Check sheet for the drawn part. Datum: minimum x, y, z corner. Units: mm. Coordinates: 2 decimals unless noted, no trailing zeros. Write each loop counter-clockwise with the first axis right and the second up, starting at its lowest first coordinate (ties: lowest second). Pieces come first, ordered by that corner, then holes. Notation, with made-up numbers: (73.5, -39.75) - (114.5, -39.75) arc R19 ccw to (114.5, -6.75) - close; hole circle Ø3 at (15, 28.25). An arc over 180 degrees is marked (long way). Write each question's results on one line, items separated by ' | '.
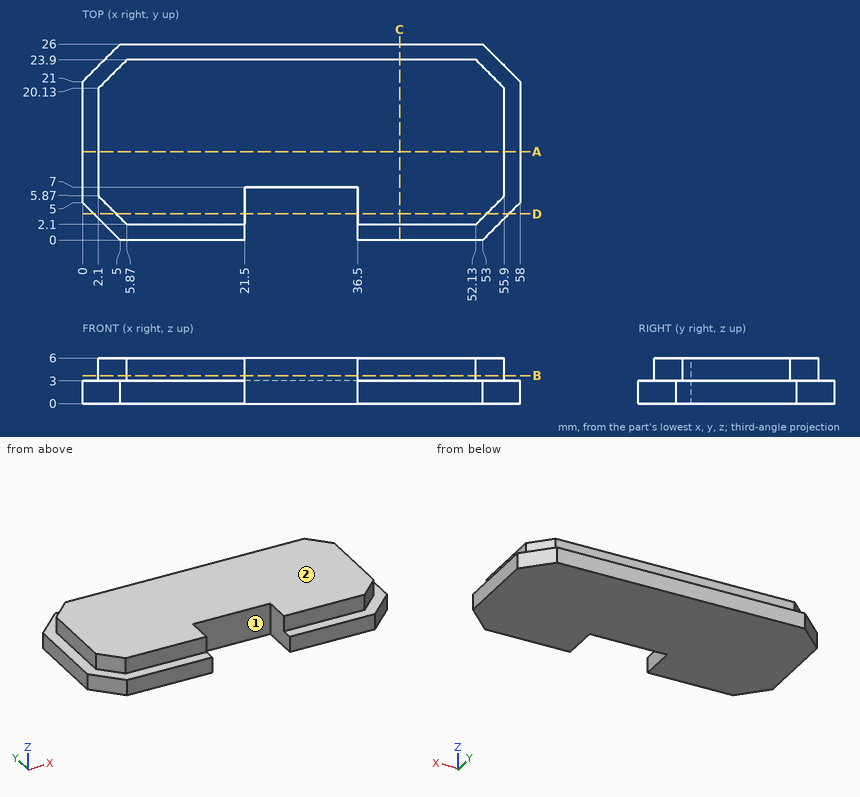
1. Draft check along X on the marked faces 1 and 2. Enter one of: pulls with the +X half, pulls with the -X half, needs draft (parallel to the pull), parting line crosses it, or undercut.
Values follow:
face 1: undercut | face 2: needs draft
2. Go/stop test with flat-tipped pins: pin 1 (0.9 mm diameter, centred on x = 23.5, z = 4, fed in from +Y); pin 2 (1 mm diameter, centred on y = 11, z = 5.5, fed in from +X); pin 3 (1.5 mm diameter, centred on y = 12.5, z = 5, fed in from -X). Record where each tip stops, or that it passes through.
Values follow:
pin 1: stops at y = 23.9 | pin 2: stops at x = 55.9 | pin 3: stops at x = 2.1
3. Sectioned sample at D-D (y = 3.5). Record the cut outline in (x, z), then the cut area to 3 significant figures.
Values follow:
outline: (1.5, 0) - (21.5, 0) - (21.5, 6) - (4.47, 6) - (4.47, 3) - (1.5, 3) - close; (36.5, 0) - (56.5, 0) - (56.5, 3) - (53.53, 3) - (53.53, 6) - (36.5, 6) - close | area: 222 mm^2
4. Material ranges on L1, parallel to X at y = 5.5, z = 2.3; L2, parallel to X at y = 14.25, z = 3.4; L3, parallel to Z at x = 8.5, y = 1.75, recorded low to high. Write a range as [from, to].
Values follow:
L1: x = [0, 21.5], [36.5, 58] | L2: x = [2.1, 55.9] | L3: z = [0, 3]
5. Sectioned sample at A-A (y = 11.75). Record the cut outline in (x, z), then the cut area to 3 significant figures.
Values follow:
outline: (0, 0) - (58, 0) - (58, 3) - (55.9, 3) - (55.9, 6) - (2.1, 6) - (2.1, 3) - (0, 3) - close | area: 335 mm^2
6. Sectioned sample at C-C (x = 42). Record the cut outline in (y, z).
Values follow:
outline: (0, 0) - (26, 0) - (26, 3) - (23.9, 3) - (23.9, 6) - (2.1, 6) - (2.1, 3) - (0, 3) - close
7. Sectioned sample at B-B (z = 3.7). Record the cut outline in (x, y).
Values follow:
outline: (2.1, 5.87) - (5.87, 2.1) - (21.5, 2.1) - (21.5, 7) - (36.5, 7) - (36.5, 2.1) - (52.13, 2.1) - (55.9, 5.87) - (55.9, 20.13) - (52.13, 23.9) - (5.87, 23.9) - (2.1, 20.13) - close
